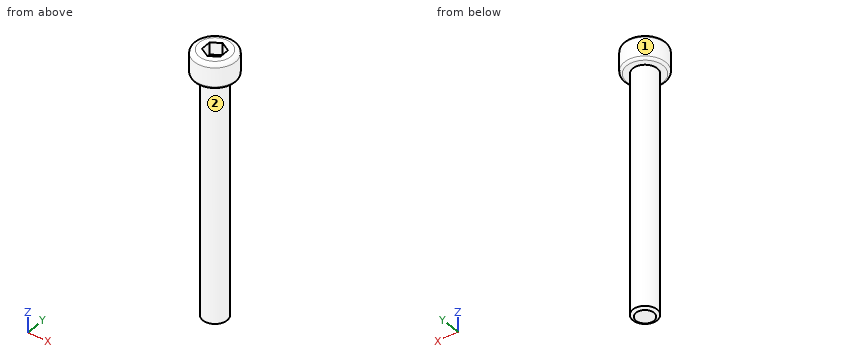
from build123d import *

# Parameters (mm, degrees)
CHAMFER_1_SIZE      = 0.3
CHAMFER_1_SIZE2     = 0.519615242
FILLET_1_R          = 0.4
FILLET_2_SIZE       = 0.5
FILLET_2_SIZE_2     = 0.8
CUT_EXTRUDE_1_DEPTH = 2


with BuildPart() as part:
    # 草图2 → 旋转1 (revolve)
    with BuildSketch(Plane(origin=(0, 0, 0), x_dir=(0, 0, -1), z_dir=(1, 0, 0)), mode=Mode.PRIVATE) as revolve_1_sk:
        Polygon((-22, 0), (-22, 3.4), (-18, 3.4), (-18, 2), (22, 2), (22, 0), align=None)
    revolve(revolve_1_sk.sketch.rotate(Axis((0, 0, -22), (0, 0, 1)), 90), axis=Axis((0, 0, -22), (0, 0, 1)))

    # 倒角1
    chamfer_1_edges = [part.edges().sort_by_distance(p)[0] for p in [
        (2, 0, -22),
    ]]
    chamfer_1_side = [part.faces().sort_by_distance(p)[0] for p in [
        (2, 0, -2),
    ]]
    chamfer(chamfer_1_edges, length=CHAMFER_1_SIZE, length2=CHAMFER_1_SIZE2, reference=chamfer_1_side[0])

    # 圆角1
    fillet_1_edges = [part.edges().sort_by_distance(p)[0] for p in [
        (3.4, 0, 18),
    ]]
    fillet(fillet_1_edges, radius=FILLET_1_R)

    # 圆角2
    # an asymmetric fillet: 0.8, 0.5 mm, written as the material it takes off along each edge
    with BuildSketch(Plane(origin=(0, 0, 22), x_dir=(-1, 0, 0), z_dir=(0, 1, 0))) as fillet_2_piece_1:
        with BuildLine():
            Bezier((3.4, -FILLET_2_SIZE), (3.4, 0), (3.4 - FILLET_2_SIZE_2, 0), weights=[1, 0.707106781, 1])
            Line((3.4 - FILLET_2_SIZE_2, 0), (3.4, 0))
            Line((3.4, 0), (3.4, -FILLET_2_SIZE))
        make_face()
    revolve(axis=Axis((0, 0, 22), (0, 0, 1)), mode=Mode.SUBTRACT)

    # 草图3 → 切除-拉伸1 (cut)
    with BuildSketch(Plane.XY.offset(22)):
        Polygon((0, 1.732050808), (-1.5, 0.866025404), (-1.5, -0.866025404), (0, -1.732050808), (1.5, -0.866025404), (1.5, 0.866025404), align=None)
    extrude(amount=-CUT_EXTRUDE_1_DEPTH, mode=Mode.SUBTRACT)


solid = part.part
Design review of the part built by this model. Coordinates are the model's own, in mm. Face numbers are marked on the shaded views. A direction names the side the tool comes from. Give positions to 0.01 mm unless a question says otherwise; leave off trailing zeros. Order: outer loops, then holes, each group sorted by start corner. A loop starts at its lowest first (then second) coordinate and runs counter-clockwise, first axis right, second up.
1. Add section B-B, the plane z = 19. State the section outline as (x, y) points.
Solution:
outline: circle Ø6.8 at (0, 0)
2. To check wall thickness, follow L1, parallel to Z at x = -0.5, y = 1.25; L2, parallel to Z at x = 2.5, y = 0; L3, parallel to X at y = -1, z = -6. State the ranges of each line that lie inside material, in increasing order.
Solution:
L1: z = -22 to 20
L2: z = 18 to 22
L3: x = -1.73 to 1.73
3. Tool access review of the marked faces 1 and 2: name each direction out of +Z, -Z, +X, -X, +Y, -Y from which nothing blocks a thin tool from reaching the whole face with its end or side.
Solution:
face 1: +Z, -Z
face 2: -Z
4. Add section A-A, the plane z = -1. State the section outline as (x, y) points, then the cut area to 3 significant figures.
Solution:
outline: circle Ø4 at (0, 0)
area: 12.6 mm2
5. For pin 1 Ø3.5 at (x, y) = (-0.5, -0.5) entering from +Z; pin 2 Ø1 at (x, y) = (-2.5, 2) entering from -Z; pin 3 Ø2 at (y, z) = (2, -9.5) entering from -X; pin 4 Ø1 at (y, z) = (0, 11.5) entering from -X, all flat-tipped, find the tip position at first contact; note any pin that passes through.
Solution:
pin 1: stops at z = 22
pin 2: stops at z = 18
pin 3: stops at x = -1.73
pin 4: stops at x = -2
